```python
from build123d import *

# Parameters (mm, degrees)
SKETCH1_R           = 2.3
SKETCH1_R_2         = 5
SKETCH1_R_3         = 8
SKETCH1_R_4         = 1.6
BOSS_EXTRUDE1_DEPTH = 3
FILLET1_R           = 3


with BuildPart() as part:
    # Sketch1 → Boss-Extrude1 (new body)
    with BuildSketch(Plane.XY):
        with BuildLine():
            Line((157.960700719, -71.866196008), (170.473892307, -71.866196008))
            ThreePointArc((170.473892307, -71.866196008), (177.544960119, -74.795128196), (180.473892307, -81.866196008))
            Line((180.473892307, -81.866196008), (180.473892307, -102.365535019))
            Line((180.473892307, -102.365535019), (180.473892307, -105.365535019))
            Line((180.473892307, -105.365535019), (170.198907285, -105.365535019))
            Line((170.198907285, -105.365535019), (170.198907285, -117.989469864))
            Line((170.198907285, -117.989469864), (180.473892307, -117.989469864))
            Line((180.473892307, -117.989469864), (180.473892307, -120.989469864))
            Line((180.473892307, -120.989469864), (180.473892307, -141.896756479))
            ThreePointArc((180.473892307, -141.896756479), (177.544960119, -148.967824291), (170.473892307, -151.896756479))
            Line((170.473892307, -151.896756479), (157.960700719, -151.896756479))
            Line((157.960700719, -151.896756479), (116.525823666, -151.896756479))
            ThreePointArc((116.525823666, -151.896756479), (109.454755854, -148.967824291), (106.525823666, -141.896756479))
            Line((106.525823666, -141.896756479), (106.525823666, -81.866196008))
            ThreePointArc((106.525823666, -81.866196008), (109.454755854, -74.795128196), (116.525823666, -71.866196008))
            Line((116.525823666, -71.866196008), (157.960700719, -71.866196008))
        make_face()
        with Locations((115.674612816, -101.866196008)):
            Circle(SKETCH1_R, mode=Mode.SUBTRACT)
        with Locations((115.674612816, -121.866196008)):
            Circle(SKETCH1_R, mode=Mode.SUBTRACT)
        with Locations((135.674612816, -141.866196008)):
            Circle(SKETCH1_R, mode=Mode.SUBTRACT)
        with Locations((135.674612816, -81.866196008)):
            Circle(SKETCH1_R, mode=Mode.SUBTRACT)
        with Locations((115.674612816, -81.866196008)):
            Circle(SKETCH1_R, mode=Mode.SUBTRACT)
        with Locations((115.674612816, -141.866196008)):
            Circle(SKETCH1_R, mode=Mode.SUBTRACT)
        with Locations((161.460700719, -96.114221831)):
            Circle(SKETCH1_R_2, mode=Mode.SUBTRACT)
        with Locations((161.460700719, -127.114221831)):
            Circle(SKETCH1_R_2, mode=Mode.SUBTRACT)
        with Locations((130.460700719, -96.114221831)):
            Circle(SKETCH1_R_2, mode=Mode.SUBTRACT)
        with Locations((145.960700719, -111.591712302)):
            Circle(SKETCH1_R_3, mode=Mode.SUBTRACT)
        with Locations((175.843347401, -96.114221831)):
            Circle(SKETCH1_R_4, mode=Mode.SUBTRACT)
        with Locations((157.960700719, -81.591712302)):
            Circle(SKETCH1_R_2, mode=Mode.SUBTRACT)
        with Locations((157.960700719, -141.591712302)):
            Circle(SKETCH1_R_2, mode=Mode.SUBTRACT)
        with Locations((175.843347401, -127.114221831)):
            Circle(SKETCH1_R_4, mode=Mode.SUBTRACT)
        with Locations((130.460700719, -127.114221831)):
            Circle(SKETCH1_R_2, mode=Mode.SUBTRACT)
    extrude(amount=BOSS_EXTRUDE1_DEPTH)

    # Fillet1
    fillet1_edges = [part.edges().sort_by_distance(p)[0] for p in [
        (180.473892307, -105.365535019, 1.5),
        (170.198907285, -105.365535019, 1.5),
        (170.198907285, -117.989469864, 1.5),
        (180.473892307, -117.989469864, 1.5),
    ]]
    fillet(fillet1_edges, radius=FILLET1_R)


solid = part.part
```
Check sheet for the modelled part. Datum: model origin and axes. Units: mm. A direction names the side the tool comes from. Round coordinates to 2 decimals unless told otherwise and drop trailing zeros. Write each loop counter-clockwise with the first axis right and the second up, starting at its lowest first coordinate (ties: lowest second). Pieces come first, ordered by that corner, then holes. Notation, with made-up numbers: (43, 13.25) -> (48, 13.25) arc R19 cw to (48, 32.25) -> close; hole circle Ø10 at (-7.75, 37.5). An arc over 180 degrees is marked (long way). Put each result on its own line as item: value.
(1) Tool access check on faces 4 (the face through (133.15, -122.9, 1.48)), 5 (the face through (179.62, -104.46, 1.52)). Record the directions out of +Z, -Z, +X, -X, +Y, -Y that give a thin tool (end or side, any length) a straight path to the whole face; none if there is none.
Values found:
face 4: +Z, -Z
face 5: +Z, -Z, +X
(2) Sectioned sample at C-C (y = -78). Enter the section's corners in (x, z), plus the area to 3 significant figures.
Values found:
outline: (107.3, 0) -> (154.48, 0) -> (154.48, 3) -> (107.3, 3) -> close; (161.44, 0) -> (179.7, 0) -> (179.7, 3) -> (161.44, 3) -> close
area: 196 mm^2
(3) Material ranges on line 1 (X direction, y = -96, z = 1.9); line 2 (Y direction, x = 135.5, z = 2.05); line 3 (Y direction, x = 128.5, z = 1.4), recorded low to high.
Values found:
line 1: x = 106.53 to 125.46, 135.46 to 156.46, 166.46 to 174.25, 177.44 to 180.47
line 2: y = -151.9 to -144.16, -139.57 to -84.16, -79.57 to -71.87
line 3: y = -151.9 to -131.71, -122.51 to -100.71, -91.51 to -71.87
(4) Go/stop test with flat-tipped pins: pin 1 Ø4 at (x, y) = (135.67, -141.87) entering from +Z; pin 2 Ø1.5 at (x, z) = (175, 2) entering from +Y. Record where each tip stops, or that it passes through.
Values found:
pin 1: passes through
pin 2: stops at y = -72.61
(5) Sectioned sample at B-B (x = 115.5). Enter the section's corners in (y, z).
Values found:
outline: (-151.84, 0) -> (-144.16, 0) -> (-144.16, 3) -> (-151.84, 3) -> close; (-139.57, 0) -> (-124.16, 0) -> (-124.16, 3) -> (-139.57, 3) -> close; (-119.57, 0) -> (-104.16, 0) -> (-104.16, 3) -> (-119.57, 3) -> close; (-99.57, 0) -> (-84.16, 0) -> (-84.16, 3) -> (-99.57, 3) -> close; (-79.57, 0) -> (-71.92, 0) -> (-71.92, 3) -> (-79.57, 3) -> close
(6) Mould release check, pull along X, two halves, no side actions. Record for faces 1 (the face through (170.199, -112, 1)), 2 (the face through (133.849, -143.266, 1.479)), 3 (the face through (175, -117.989, 1)): released by +X, released by -X, zero draft, split by the parting line, or undercut.
Values found:
face 1: released by +X
face 2: undercut
face 3: zero draft
(7) Sectioned sample at D-D (x = 130). Enter the section's corners in (y, z), plus the area to 3 significant figures.
Values found:
outline: (-151.9, 0) -> (-132.09, 0) -> (-132.09, 3) -> (-151.9, 3) -> close; (-122.14, 0) -> (-101.09, 0) -> (-101.09, 3) -> (-122.14, 3) -> close; (-91.14, 0) -> (-71.87, 0) -> (-71.87, 3) -> (-91.14, 3) -> close
area: 180 mm^2
(8) Sectioned sample at A-A (x = 147). Enter the section's corners in (y, z).
Values found:
outline: (-151.9, 0) -> (-119.52, 0) -> (-119.52, 3) -> (-151.9, 3) -> close; (-103.66, 0) -> (-71.87, 0) -> (-71.87, 3) -> (-103.66, 3) -> close
